Part model, mm, in its own coordinate system. A direction names the side the tool comes from. Coordinates: 2 decimals unless noted, no trailing zeros. Write each loop counter-clockwise with the first axis right and the second up, starting at its lowest first coordinate (ties: lowest second). Pieces come first, ordered by that corner, then holes. Notation, with made-up numbers: M -23,45 L -8,45 A7 ccw -8,55 Z; hole C 82,25.25 d1. An arc over 180 degrees is marked long. Use a Markdown table: item, result. Add a question column.
Q1. Pin check, flat tips, straight feed: pin 1 Ø1.5 at (x, z) = (-6.5, -35.5) entering from -Y; pin 2 Ø3 at (x, z) = (28.5, -33.25) entering from -Y; pin 3 Ø10 at (y, z) = (18.5, -57) entering from +X. Stop position of each tip, or through.
Q2. Mould opens along Z. For faces 3 (the flat face through (29, 30, -1)), 4 (the flat face through (0, 25, -50)), 5 (the flat face through (-5, 30, 40)), 6 (the flat face through (4, 25, 100)) say: released by +Z, released by -Z, zero draft, split by the parting line, or undercut.
Q3. Tool access for faces 1 (the flat face through (25, 22, 1)), 2 (the flat face through (-5, 30, 85)): list every direction of +Z, -Z, +X, -X, +Y, -Y with a clear straight run to the whole face (end or side of a thin tool).
Q4. Slice it at B-B on x = 21. Write the cut outline in (y, z), then the cut area to 3 significant figures.
Q5. Slice it at D-D on y = 31.75. Count the separate pieces of the cut face and the enclosed holes in it, then the cut area to 3 significant figures.
Q6. Wall check: L1, parallel to X at y = 31.2, z = -33.25; L2, parallel to Z at x = 1.5, y = 17.5; L3, parallel to X at y = 26.25, z = 78.5. Give the ranges that are in metal, low to high. Write a range as from..to.
Q7. Slice it at A-A on z = -43.5. Write the cut outline in (x, y), then the cut area to 3 significant figures.
Q8. Slice it at C-C on z = 56.5. Write the cut outline in (x, y).
Autodesk Inventor part; units mm, degrees
ref_plane "YZ Plane" through (0, 0, 0) normal (1, 0, 0) x (0, 1, 0)
ref_plane "XZ Plane" through (0, 0, 0) normal (0, 1, 0) x (-1, 0, 0)
ref_plane "XY Plane" through (0, 0, 0) normal (0, 0, 1) x (1, 0, 0)
sketch "Sketch1" plane through (0, 0, 0) normal (0, 1, 0) x (-1, 0, 0)
  line L0 (-25, -100) -> (25, -100)
  line L1 (25, -100) -> (25, 100)
  line L2 (25, 100) -> (-25, 100)
  line L3 (-25, 100) -> (-25, -100)
  line L4 (-25, -100) -> (25, 100) construction
  line L5 (25, -100) -> (-25, 100) construction
  line L6 (23, 50) -> (-23, 50)
  line L7 (-23, 50) -> (-23, 30)
  line L8 (-23, 30) -> (23, 30)
  line L9 (23, 30) -> (23, 50)
  line L10 (23, 50) -> (-23, 30) construction
  line L11 (-23, 50) -> (23, 30) construction
  line L12 (23, -30) -> (-23, -30)
  line L13 (-23, -30) -> (-23, -50)
  line L14 (-23, -50) -> (23, -50)
  line L15 (23, -50) -> (23, -30)
  line L16 (23, -30) -> (-23, -50) construction
  line L17 (-23, -30) -> (23, -50) construction
  line L18 (-23, 10) -> (23, 10)
  line L19 (23, 10) -> (23, -10)
  line L20 (23, -10) -> (-23, -10)
  line L21 (-23, -10) -> (-23, 10)
  line L22 (-23, 10) -> (23, -10) construction
  line L23 (23, 10) -> (-23, -10) construction
  line L24 (-23, 95) -> (23, 95)
  line L25 (23, 95) -> (23, 75)
  line L26 (23, 75) -> (-23, 75)
  line L27 (-23, 75) -> (-23, 95)
  line L28 (-23, 95) -> (23, 75) construction
  line L29 (23, 95) -> (-23, 75) construction
  line L30 (-23, -75) -> (23, -75)
  line L31 (23, -75) -> (23, -95)
  line L32 (23, -95) -> (-23, -95)
  line L33 (-23, -95) -> (-23, -75)
  line L34 (-23, -75) -> (23, -95) construction
  line L35 (23, -75) -> (-23, -95) construction
  point P0 (0, 0)
  point P1 (0, 40)
  point P2 (0, -40)
  point P3 (0, 0)
  point P4 (0, 85)
  point P5 (0, -85)
  dimension "d0" = 200
  dimension "d1" = 50
  dimension "d2" = 2
  dimension "d3" = 46
  dimension "d4" = 20
  dimension "d5" = 46
  dimension "d6" = 20
  dimension "d7" = 2
  dimension "d8" = 20
  dimension "d9" = 46
  dimension "d10" = 2
  dimension "d11" = 0
  dimension "d12" = 20
  dimension "d13" = 20
  dimension "d14" = 46
  dimension "d15" = 20
  dimension "d16" = 20
  dimension "d17" = 46
  dimension "d18" = 2
  dimension "d19" = 2
  dimension "d20" = 25
  dimension "d21" = 25
extrude "Extrusion1" add sketch "Sketch1" along normal blind 35
sketch "Sketch2" plane through (0, 35, 0) normal (0, 1, 0) x (1, 0, 0)
  line L0 (23, -95) -> (-23, -95)
  line L1 (-23, -75) -> (23, -75)
  line L2 (-8, -95) -> (-5, -95)
  line L3 (-5, -95) -> (-5, -75)
  line L4 (-5, -75) -> (-8, -75)
  line L5 (-8, -75) -> (-8, -95)
  line L6 (-23, -30) -> (23, -30)
  line L7 (-8, -50.2373) -> (-5, -50.2373)
  line L8 (-5, -50.2373) -> (-5, -30)
  line L9 (-5, -30) -> (-8, -30)
  line L10 (-8, -30) -> (-8, -50.2373)
  line L11 (-8, -10.1346) -> (-5, -10.1346)
  line L12 (-5, -10.1346) -> (-5, 9.9167)
  line L13 (-5, 9.9167) -> (-8, 9.9167)
  line L14 (-8, 9.9167) -> (-8, -10.1346)
  line L15 (-23, 50) -> (23, 50)
  line L16 (-8, 29.7501) -> (-5, 29.7501)
  line L17 (-5, 29.7501) -> (-5, 50)
  line L18 (-5, 50) -> (-8, 50)
  line L19 (-8, 50) -> (-8, 29.7501)
  line L20 (23, 75) -> (-23, 75)
  line L21 (-23, 95) -> (23, 95)
  line L22 (-8, 75) -> (-5, 75)
  line L23 (-5, 75) -> (-5, 95)
  line L24 (-5, 95) -> (-8, 95)
  line L25 (-8, 95) -> (-8, 75)
  line L26 (-23, -95) -> (-23, -75)
  line L27 (-23, 75) -> (-23, 95)
  point P0 (0, 0)
  dimension "d24" = 3
  dimension "d25" = 3
  dimension "d26" = 3
  dimension "d27" = 3
  dimension "d28" = 3
  dimension "d29" = 15
  dimension "d30" = 15
extrude "Extrusion2" add sketch "Sketch2" against normal blind 10 contours L0 L5 L1 L3 | L6 L8 L7 L10 | L14 L13 L12 L11 | L15 L17 L16 L19 | L20 L25 L21 L23
sketch "Sketch3" plane through (0, 35, 0) normal (0, 1, 0) x (1, 0, 0)
  line L0 (-5, -10) -> (-5, 9.9167)
  line L1 (-8, 30) -> (-8, 50)
  line L2 (-5, 8.437) -> (-8, 8.437)
  line L3 (-8, 8.437) -> (-8, 32.4131)
  line L4 (-8, 32.4131) -> (-5, 32.4131)
  line L5 (-5, 32.4131) -> (-5, 8.437)
  point P0 (0, 0)
extrude "Extrusion3" add sketch "Sketch3" against normal blind 10
sketch "Sketch4" plane through (25, 0, -100) normal (0, 0, -1) x (-1, 0, 0)
  line L0 (0, 35) -> (-7, 35)
  line L1 (-7, 35) -> (-7, 30)
  line L2 (-7, 30) -> (0, 30)
  line L3 (0, 30) -> (0, 35)
  line L4 (0, 0) -> (0, 35)
  line L5 (0, 35) -> (50, 35)
  point P0 (25, 0)
  dimension "d35" = 0
  dimension "d36" = 7
  dimension "d37" = 5
  dimension "d38" = 0
extrude "Extrusion4" add sketch "Sketch4" against normal blind 200
sketch "Sketch5" plane through (25, 0, -100) normal (0, 0, -1) x (-1, 0, 0)
  point P0 (25, 0)
sketch "Sketch6" plane through (0, 35, 0) normal (0, 1, 0) x (1, 0, 0)
  circle A0 centre (28.5, -33.25) radius 1.25
  circle A1 centre (28.5, -26.75) radius 1.25
  line L0 (32, 100) -> (32, -100)
  circle A2 centre (28.5, -3.25) radius 1.25
  circle A3 centre (28.5, 3.25) radius 1.25
  circle A4 centre (28.5, 26.75) radius 1.25
  circle A5 centre (28.5, 33.25) radius 1.25
  line L1 (-25, 100) -> (32, 100)
  line L2 (-25, -100) -> (32, -100)
  point P0 (0, 0)
  dimension "d41" = 2.5
  dimension "d42" = 2.5
  dimension "d46" = 2.5
  dimension "d47" = 2.5
  dimension "d48" = 2.5
  dimension "d49" = 2.5
  dimension "d51" = 4
  dimension "d53" = 4
  dimension "d54" = 3.5
  dimension "d55" = 3.5
  dimension "d56" = 3.5
  dimension "d57" = 4
  dimension "d58" = 3.5
  dimension "d59" = 3.5
  dimension "d62" = 96.75
  dimension "d63" = 3.5
  dimension "d66" = 21
  dimension "d67" = 21
extrude "Extrusion5" cut sketch "Sketch6" against normal blind 30
sketch "Sketch7" plane through (25, 0, -100) normal (0, 0, -1) x (-1, 0, 0)
  point P0 (25, 0)
sketch "Sketch8" plane through (0, 35, 0) normal (0, 1, 0) x (1, 0, 0)
  point P0 (0, 0)
sketch "Sketch9" plane through (25, 0, 100) normal (1, 0, 0) x (0, 0, -1)
  line L0 (-3.3992, 0) -> (201.6008, 0)
  line L1 (201.6008, 0) -> (201.6008, 15)
  line L2 (201.6008, 15) -> (-3.3992, 15)
  line L3 (-3.3992, 15) -> (-3.3992, 0)
  line L4 (0, 0) -> (200, 0)
  point P0 (100, 0)
  dimension "d68" = 15
  dimension "d69" = 0
  dimension "d70" = 205
extrude "Extrusion6" cut sketch "Sketch9" against normal blind 55
properties part number "Fem_Sensor_Indtil_Videre"
Recorded:
| question | item | result |
|---|---|---|
| 1 | pin 1 | y = 25 |
| 1 | pin 2 | y = 30 |
| 1 | pin 3 | x = 25 |
| 2 | face 3 | zero draft |
| 2 | face 4 | undercut |
| 2 | face 5 | undercut |
| 2 | face 6 | released by +Z |
| 3 | face 1 | +Z, -Z, +X, -Y |
| 3 | face 2 | +Y, -Y |
| 4 | outline | M 15,-100 L 35,-100 L 35,-95 L 15,-95 Z; M 15,-75 L 35,-75 L 35,-50 L 15,-50 Z; M 15,-30 L 35,-30 L 35,-10 L 15,-10 Z; M 15,10 L 35,10 L 35,30 L 15,30 Z; M 15,50 L 35,50 L 35,75 L 15,75 Z; M 15,95 L 35,95 L 35,100 L 15,100 Z |
| 4 | area | 2,000 mm² |
| 5 | separate pieces | 1 |
| 5 | enclosed holes | 16 |
| 5 | area | 7,070 mm² |
| 6 | L1 | -25..-23, -8..-5, 23..27.25, 29.75..32 |
| 6 | L2 | -100..-95, -75..-50, -30..-10, 10..30, 50..75, 95..100 |
| 6 | L3 | -25..-23, -8..-5, 23..25 |
| 7 | outline | M -25,15 L -23,15 L -23,35 L -25,35 Z; M -8,25 L -5,25 L -5,35 L -8,35 Z; M 23,15 L 25,15 L 25,30 L 32,30 L 32,35 L 23,35 Z |
| 7 | area | 145 mm² |
| 8 | outline | M -25,15 L 25,15 L 25,30 L 32,30 L 32,35 L -25,35 Z |
